Here's how the part is built. I have some questions about the finished solid (model axes, mm). Face numbers are marked on the shaded views. A direction names the side the tool comes from. Coordinates: 2 decimals unless noted, no trailing zeros. Write each loop counter-clockwise with the first axis right and the second up, starting at its lowest first coordinate (ties: lowest second). Pieces come first, ordered by that corner, then holes.
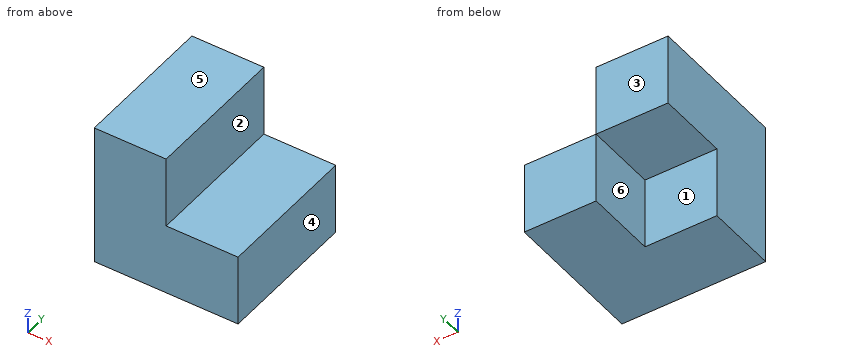
from build123d import *

# Parameters (mm, degrees)
F0_W     = 25.4
F0_H     = 25.4
F1_DEPTH = 25.4
F2_DEPTH = 50.8
F3_DEPTH = 25.3746


with BuildPart() as f1:
    # F0 (on Top) → F1 (new body)
    with BuildSketch(Plane.XY):
        with Locations((12.7, 12.7)):
            Rectangle(F0_W, F0_H)
        Polygon((25.4, 25.4), (25.4, 0), (50.8, 0), (50.8, 50.8), (25.4, 50.8), align=None)
        with Locations((12.7, 38.1)):
            Rectangle(F0_W, F0_H)
    extrude(amount=F1_DEPTH)

    # F0 (on Top) → F2 (join)
    with BuildSketch(Plane.XY):
        with Locations((12.7, 38.1)):
            Rectangle(F0_W, F0_H)
        with Locations((12.7, 12.7)):
            Rectangle(F0_W, F0_H)
    extrude(amount=F2_DEPTH)

    # F0 (on Top) → F3 (cut)
    with BuildSketch(Plane.XY):
        with Locations((12.7, 38.1)):
            Rectangle(F0_W, F0_H)
    extrude(amount=F3_DEPTH, mode=Mode.SUBTRACT)


solid = f1.part
1. I want a section at A-A (y = 47.5). List the corners of the cut face in (x, z) for me, then the cut area to 3 significant figures.
2. I want a section at C-C (x = 21.5). List the corners of the cut face in (y, z) for me, then the cut area to 3 significant figures.
3. For pin 1 Ø7.5 at (y, z) = (32.5, 38) entering from +X; pin 2 Ø5 at (y, z) = (36.5, 8) entering from -X; pin 3 Ø12.5 at (x, y) = (11, 40.5) entering from -Z; pin 4 Ø1 at (x, z) = (38.5, 27.5) entering from -Y, each with a flat end and sliding along its axis, tell me the tip position at first contact or that it passes through.
4. I want a section at D-D (x = 34). List the corners of the cut face in (y, z) for me.
5. Thinking about a two-plate mould opening in X: for the marked faces 4, 5 and 6, which applies, pulls with the +X half, pulls with the -X half, needs draft (parallel to the pull), parting line crosses it, or undercut?
6. If I drill on line 1 (X direction, y = 37.5, z = 15); line 2 (Z direction, x = 42, y = 5.5), over which ranges is the centre line in solid material (lowest first)?
7. I want a section at B-B (z = 21). List the corners of the cut face in (x, y) for me, then the cut area to 3 significant figures.
8. On a 3-axis mill with a long thin cutter (end or side, diameter ignored), from which of +Z, -Z, +X, -X, +Y, -Y can I reach the whole of each face in a straight line? I mean the marked faces 1, 2 and 3. Say none if no direction works.
Response values:
1. outline: (0, 25.37) - (25.4, 25.37) - (25.4, 0) - (50.8, 0) - (50.8, 25.4) - (25.4, 25.4) - (25.4, 50.8) - (0, 50.8) - close
1. area: 1,290 mm2
2. outline: (0, 0) - (25.4, 0) - (25.4, 25.37) - (50.8, 25.37) - (50.8, 50.8) - (0, 50.8) - close
2. area: 1,940 mm2
3. pin 1: stops at x = 25.4
3. pin 2: stops at x = 25.4
3. pin 3: stops at z = 25.37
3. pin 4: passes through
4. outline: (0, 0) - (50.8, 0) - (50.8, 25.4) - (0, 25.4) - close
5. face 4: pulls with the +X half
5. face 5: needs draft
5. face 6: pulls with the -X half
6. line 1: x = 25.4 to 50.8
6. line 2: z = 0 to 25.4
7. outline: (0, 0) - (50.8, 0) - (50.8, 50.8) - (25.4, 50.8) - (25.4, 25.4) - (0, 25.4) - close
7. area: 1,940 mm2
8. face 1: -Z, -X, +Y
8. face 2: +Z, +X, +Y, -Y
8. face 3: +Z, -Z, +X, -X, +Y
